Work out the finished part from the listing and answer in its coordinate system (mm). A direction names the side the tool comes from. Give positions to 0.01 mm unless a question says otherwise; leave off trailing zeros. Write each loop counter-clockwise with the first axis right and the second up, starting at its lowest first coordinate (ties: lowest second). Pieces come first, ordered by that corner, then holes. Notation, with made-up numbers: (87, -25) - (102, -25) arc R18 cw to (102, 1) - close; hole circle Ø8 at (-15.75, 12.25). An arc over 180 degrees is marked (long way). Write item = value, one per line.
from build123d import *

# Parameters (mm, degrees)
SKICA1_W                 = 26
SKICA1_H                 = 1
P_IDAT_VYSUNUT_M1_DEPTH  = 10
SKICA2_R                 = 2.5
ODEBRAT_VYSUNUT_M1_DEPTH = 1
SKICA3_R                 = 2.4
P_IDAT_VYSUNUT_M2_DEPTH  = 0.8
SKICA4_W                 = 26
SKICA4_H                 = 10
SKICA4_R                 = 3
P_IDAT_VYSUNUT_M3_DEPTH  = 1.2
SKICA6_W                 = 8
SKICA6_H                 = 0.7
P_IDAT_VYSUNUT_M5_DEPTH  = 9
P_IDAT_VYSUNUT_M6_DEPTH  = 8
P_IDAT_VYSUNUT_M8_DEPTH  = 0.7
P_IDAT_VYSUNUT_M9_DEPTH  = 0.7


with BuildPart() as part:
    # Skica1 → Přidat vysunutím1 (new body)
    with BuildSketch(Plane.XY):
        with Locations((-39.156744291, -7.214704976)):
            Rectangle(SKICA1_W, SKICA1_H)
    extrude(amount=P_IDAT_VYSUNUT_M1_DEPTH)

    # Skica2 → Odebrat vysunutím1 (cut)
    with BuildSketch(Plane(origin=(0, -7.714704976, 0), x_dir=(-1, 0, 0), z_dir=(0, -1, 0))):
        with Locations((48.186744291, -5)):
            Circle(SKICA2_R)
        with Locations((42.176744291, -5)):
            Circle(SKICA2_R)
        with Locations((36.166744291, -5)):
            Circle(SKICA2_R)
        with Locations((30.156744291, -5)):
            Circle(SKICA2_R)
    extrude(amount=-ODEBRAT_VYSUNUT_M1_DEPTH, mode=Mode.SUBTRACT)

    # Skica3 → Přidat vysunutím2 (add)
    with BuildSketch(Plane(origin=(0, -6.714704976, 0), x_dir=(1, 0, 0), z_dir=(0, 1, 0))):
        Polygon((-32.956744291, 0), (-18.656744291, 15.3), (-18.656744291, 22.3), (-11.856744291, 22.3), (-11.856744291, 15.3), (-26.156744291, 0), align=None)
        with Locations((-15.756744291, 18.4)):
            Circle(SKICA3_R, mode=Mode.SUBTRACT)
        Polygon((-52.156744291, 0), (-45.356744291, 0), (-59.656744291, 15.3), (-59.656744291, 22.3), (-66.456744291, 22.3), (-66.456744291, 15.3), align=None)
        with Locations((-62.556744291, 18.4)):
            Circle(SKICA3_R, mode=Mode.SUBTRACT)
        Polygon((-45.356744291, -10), (-59.656744291, -25.3), (-59.656744291, -32.3), (-66.456744291, -32.3), (-66.456744291, -25.3), (-52.156744291, -10), align=None)
        with Locations((-62.556744291, -28.4)):
            Circle(SKICA3_R, mode=Mode.SUBTRACT)
        Polygon((-26.156744291, -10), (-32.956744291, -10), (-18.656744291, -25.3), (-18.656744291, -32.3), (-11.856744291, -32.3), (-11.856744291, -25.3), align=None)
        with Locations((-15.756744291, -28.4)):
            Circle(SKICA3_R, mode=Mode.SUBTRACT)
    extrude(amount=-P_IDAT_VYSUNUT_M2_DEPTH)

    # Skica4 → Přidat vysunutím3 (add)
    with BuildSketch(Plane(origin=(0, -7.714704976, 0), x_dir=(-1, 0, 0), z_dir=(0, -1, 0))):
        with Locations((39.156744291, -5)):
            Rectangle(SKICA4_W, SKICA4_H)
        with Locations((48.186744291, -5)):
            Circle(SKICA4_R, mode=Mode.SUBTRACT)
        with Locations((42.176744291, -5)):
            Circle(SKICA4_R, mode=Mode.SUBTRACT)
        with Locations((36.166744291, -5)):
            Circle(SKICA4_R, mode=Mode.SUBTRACT)
        with Locations((30.156744291, -5)):
            Circle(SKICA4_R, mode=Mode.SUBTRACT)
    extrude(amount=P_IDAT_VYSUNUT_M3_DEPTH)

    # Skica6 → Přidat vysunutím5 (add)
    with BuildSketch(Plane(origin=(0, -6.714704976, 0), x_dir=(1, 0, 0), z_dir=(0, 1, 0))):
        with Locations((-39.156744291, 0.35)):
            Rectangle(SKICA6_W, SKICA6_H)
        with Locations((-39.156744291, -10.35)):
            Rectangle(SKICA6_W, SKICA6_H)
    extrude(amount=-P_IDAT_VYSUNUT_M5_DEPTH)

    # Skica7 → Přidat vysunutím6 (add)
    with BuildSketch(Plane(origin=(-35.156744291, 0, 0), x_dir=(0, 0, -1), z_dir=(1, 0, 0))):
        Polygon((-10, -15.714704976), (-9.5, -15.714704976), (-10, -15.214704976), align=None)
        Polygon((0, -15.714704976), (0, -15.214704976), (-0.5, -15.714704976), align=None)
    extrude(amount=-P_IDAT_VYSUNUT_M6_DEPTH)

    # Skica8 → Přidat vysunutím8 (add)
    with BuildSketch(Plane(origin=(0, 0, 0), x_dir=(-1, 0, 0), z_dir=(0, 0, -1))):
        Polygon((43.156744291, -6.714704976), (43.156744291, -10.714704976), (47.156744291, -6.714704976), align=None)
        Polygon((35.156744291, -10.714704976), (35.156744291, -6.714704976), (31.156744291, -6.714704976), align=None)
    extrude(amount=P_IDAT_VYSUNUT_M8_DEPTH)

    # Skica9 → Přidat vysunutím9 (add)
    with BuildSketch(Plane.XY.offset(10)):
        Polygon((-43.156744291, -6.714704976), (-47.156744291, -6.714704976), (-43.156744291, -10.714704976), align=None)
        Polygon((-35.156744291, -6.714704976), (-35.156744291, -10.714704976), (-31.156744291, -6.714704976), align=None)
    extrude(amount=P_IDAT_VYSUNUT_M9_DEPTH)


solid = part.part
1. Given pin 1 (0.7 mm diameter, centred on y = -7.5, z = 7.5, fed in from -X); pin 2 (9.5 mm diameter, centred on x = -48.19, z = 5, fed in from -Y); pin 3 (7.5 mm diameter, centred on x = -62.56, z = -18.4, fed in from -Y), each flat-ended and moving along its own axis, determine where each tip first touches the part or whether it passes through.
Solution:
pin_1 = -52.16
pin_2 = -8.91
pin_3 = -7.51
2. Straight lines are drawn through the part: line 1 (X direction, y = -7.2, z = 28.4); line 2 (Z direction, x = -36, y = -8); line 3 (X direction, y = -7.1, z = 5). For each, find the intervals that lie inside material, in ascending order.
Solution:
line_1 = -66.46 to -64.96, -60.16 to -59.66, -18.66 to -18.16, -13.36 to -11.86
line_2 = -0.7 to 2, 8 to 10.7
line_3 = -52.16 to -50.69, -45.69 to -44.68, -39.68 to -38.67, -33.67 to -32.66, -27.66 to -26.16
3. Find section A-A, the plane y = -12.5. Give the vertices of the cut face in (x, z), then the cut area to 3 significant figures.
Solution:
outline = (-43.16, -0.7) - (-35.16, -0.7) - (-35.16, 0) - (-43.16, 0) - close; (-43.16, 10) - (-35.16, 10) - (-35.16, 10.7) - (-43.16, 10.7) - close
area = 11.2 mm^2
4. Find section B-B, the plane z = -18.4. Give the vertices of the cut face in (x, y).
Solution:
outline = (-66.46, -7.51) - (-64.96, -7.51) - (-64.96, -6.71) - (-66.46, -6.71) - close; (-60.16, -7.51) - (-59.66, -7.51) - (-59.66, -6.71) - (-60.16, -6.71) - close; (-18.66, -7.51) - (-18.16, -7.51) - (-18.16, -6.71) - (-18.66, -6.71) - close; (-13.36, -7.51) - (-11.86, -7.51) - (-11.86, -6.71) - (-13.36, -6.71) - close
5. For a pull along Y with two mould halves and no side action, classify faces 4 (the flat face through (-39, -12, 0)), 5 (the flat face through (-21, -7.515, 19)), 6 (the flat face through (-59.41, -7.11, 17.76)) as pulls with the +Y half, pulls with the -Y half, needs draft (parallel to the pull), parting line crosses it, or undercut.
Solution:
face_4 = undercut
face_5 = pulls with the -Y half
face_6 = needs draft
6. Find section C-C, the plane z = 15. Give the vertices of the cut face in (x, y), then the cut area to 3 significant figures.
Solution:
outline = (-56.83, -7.51) - (-50.03, -7.51) - (-50.03, -6.71) - (-56.83, -6.71) - close; (-28.28, -7.51) - (-21.48, -7.51) - (-21.48, -6.71) - (-28.28, -6.71) - close
area = 10.9 mm^2
7. A tool of negligible diameter and unlimited length cuts with its end or side. For faces 1 (the flat face through (-44.78, -9.09, 10.35)), 2 (the cylindrical face through (-39.97, -8.31, 2.97)), 3 (the flat face through (-18.907, -7.109, -7.757)), from which of +Z, -Z, +X, -X, +Y, -Y can it reach the whole face along a straight path? Write none if from no direction.
Solution:
face_1 = +Z, -X, -Y
face_2 = -Y
face_3 = +X, +Y, -Y
8. Find section D-D, the plane z = 5. Give the number of separate pieces and of enclosed holes in the cut face, then the cut area to 3 significant figures.
Solution:
separate_pieces = 5
enclosed_holes = 0
area = 8.40 mm^2
